Geometry check sheet. Reference: the model listing, model coordinates, mm. Round coordinates to 2 decimals unless told otherwise and drop trailing zeros. Order: outer loops, then holes, each group sorted by start corner. A loop starts at its lowest first (then second) coordinate and runs counter-clockwise, first axis right, second up.
```python
from build123d import *

# Parameters (mm, degrees)
SKETCH001_R        = 1.5
POCKET_DEPTH       = 25.505705
POCKET_DEPTH_BACK  = 27.555705
POLARPATTERN_COUNT = 2


with BuildPart() as part:
    # Sketch → Revolution (revolve)
    with BuildSketch(Plane.XZ):
        Polygon((2.4, 0), (4.45, 0), (2.4, 2.05), align=None)
    revolve(axis=Axis((0, 0, 0), (0, 0, 1)))

    # Sketch001 → Pocket (cut, two sides)
    with BuildSketch(Plane.XY) as pocket_sk:
        with Locations((0, 5)):
            Circle(SKETCH001_R)
    pocket = extrude(amount=-POCKET_DEPTH, mode=Mode.SUBTRACT) + extrude(pocket_sk.sketch, amount=POCKET_DEPTH_BACK, mode=Mode.SUBTRACT)

    # PolarPattern: Pocket ×2 about axis
    polarpattern_axis = Axis((0, 0, 0), (0, 0, 1))
    for i in range(1, POLARPATTERN_COUNT):
        add(pocket.rotate(polarpattern_axis, i * 360 / POLARPATTERN_COUNT), mode=Mode.SUBTRACT)


solid = part.part
```
(1) Sectioned sample at D-D, the plane z = 1.95. Record the cut outline in (x, y), and give its area (3 significant figures).
Returned:
outline: circle Ø5 at (0, 0); hole circle Ø4.8 at (0, 0)
area: 1.54 mm2
(2) Sectioned sample at A-A, the plane x = 0. Record the cut outline in (y, z), and give its area (3 significant figures).
Returned:
outline: (-3.5, 0) - (-2.4, 0) - (-2.4, 2.05) - (-3.5, 0.95) - close; (2.4, 0) - (3.5, 0) - (3.5, 0.95) - (2.4, 2.05) - close
area: 3.30 mm2
(3) Draft check along Y on faces 1 (the cylindrical face through (1.29, 2.024, 1.011)), 2 (the cylindrical face through (0, -3.5, 0.4)), 3 (the flat face through (-2, -2, 0)). Enter one of: released by +Y, released by -Y, zero draft, split by the parting line, or undercut.
Returned:
face 1: undercut
face 2: released by -Y
face 3: zero draft
(4) Depth check by flat-ended pin: P1, Ø1, axis at y = 2, z = 1, coming from the -X side. Enter the tip coordinate at first touch or a pass-through.
Returned:
P1: stops at x = -3.47
(5) Material ranges on line 1 (Y direction, x = 0, z = 0.65); line 2 (X direction, y = 1.25, z = 1); line 3 (Y direction, x = 0, z = 1.3), recorded low to high.
Returned:
line 1: y = -3.5 to -2.4, 2.4 to 3.5
line 2: x = -3.22 to -2.05, 2.05 to 3.22
line 3: y = -3.15 to -2.4, 2.4 to 3.15
(6) Sectioned sample at B-B, the plane y = 0. Record the cut outline in (x, z).
Returned:
outline: (-4.45, 0) - (-2.4, 0) - (-2.4, 2.05) - close; (2.4, 0) - (4.45, 0) - (2.4, 2.05) - close
(7) Sectioned sample at C-C, the plane z = 0.6. Record the cut outline in (x, y), and give its area (3 significant figures).
Returned:
outline: (-0.84, -3.76) arc R1.5 cw to (0.84, -3.76) arc R3.85 ccw to (0.84, 3.76) arc R1.5 cw to (-0.84, 3.76) arc R3.85 ccw to start; hole circle Ø4.8 at (0, 0)
area: 27.7 mm2
